Could you check a few things on this model? Use its own coordinates, in mm. Face numbers are marked on the shaded views. A direction names the side the tool comes from. Round coordinates to 2 decimals unless told otherwise and drop trailing zeros. Loops run counter-clockwise (first coordinate to the right, second up) from the corner with the lowest first, then second, coordinate; pieces in that order, holes last. Notation, with made-up numbers: (40, 34.5) -> (72, 34.5) arc R26 ccw to (72, 71.5) -> close; hole circle Ø3 at (-27.5, 77). An arc over 180 degrees is marked (long way). One line per item, written item: value.
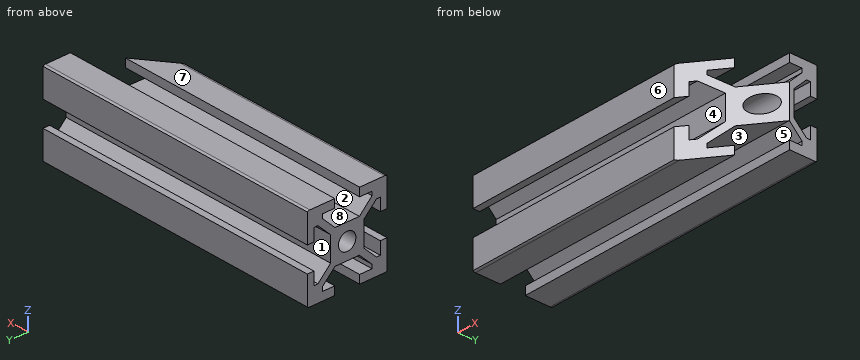
```python
from build123d import *

# Parameters (mm, degrees)
SKETCH1_R                = 2.1
BOSS_EXTRUDE1_DEPTH      = 70
CUT_EXTRUDE_1_DEPTH      = 1
CUT_EXTRUDE_1_DEPTH_BACK = 21


with BuildPart() as part:
    # Sketch1 → Boss-Extrude1 (new body)
    with BuildSketch(Plane(origin=(0, 0, 0), x_dir=(0, 0, -1), z_dir=(1, 0, 0))):
        with BuildLine():
            Line((-10, 9), (-10, 3))
            Line((-10, 3), (-8, 3))
            Line((-8, 3), (-8, 6))
            Line((-8, 6), (-7.060660172, 6))
            Line((-7.060660172, 6), (-4, 2.939339828))
            Line((-4, 2.939339828), (-4, -2.939339828))
            Line((-4, -2.939339828), (-7.060660172, -6))
            Line((-7.060660172, -6), (-8, -6))
            Line((-8, -6), (-8, -3))
            Line((-8, -3), (-10, -3))
            Line((-10, -3), (-10, -9))
            ThreePointArc((-10, -9), (-9.948683298, -9.316227766), (-9.8, -9.6))
            Line((-9.8, -9.6), (-3, -9.6))
            Line((-3, -9.6), (-3, -8))
            Line((-3, -8), (-6, -8))
            Line((-6, -8), (-6, -7.060660172))
            Line((-6, -7.060660172), (-2.939339828, -4))
            Line((-2.939339828, -4), (2.939339828, -4))
            Line((2.939339828, -4), (6, -7.060660172))
            Line((6, -7.060660172), (6, -8))
            Line((6, -8), (3, -8))
            Line((3, -8), (3, -9.6))
            Line((3, -9.6), (9.8, -9.6))
            ThreePointArc((9.8, -9.6), (9.948683298, -9.316227766), (10, -9))
            Line((10, -9), (10, -3))
            Line((10, -3), (8, -3))
            Line((8, -3), (8, -6))
            Line((8, -6), (7.060660172, -6))
            Line((7.060660172, -6), (4, -2.939339828))
            Line((4, -2.939339828), (4, 2.939339828))
            Line((4, 2.939339828), (7.060660172, 6))
            Line((7.060660172, 6), (8, 6))
            Line((8, 6), (8, 3))
            Line((8, 3), (10, 3))
            Line((10, 3), (10, 9))
            ThreePointArc((10, 9), (9.948683298, 9.316227766), (9.8, 9.6))
            Line((9.8, 9.6), (3, 9.6))
            Line((3, 9.6), (3, 8))
            Line((3, 8), (6, 8))
            Line((6, 8), (6, 7.060660172))
            Line((6, 7.060660172), (2.939339828, 4))
            Line((2.939339828, 4), (-2.939339828, 4))
            Line((-2.939339828, 4), (-6, 7.060660172))
            Line((-6, 7.060660172), (-6, 8))
            Line((-6, 8), (-3, 8))
            Line((-3, 8), (-3, 9.6))
            Line((-3, 9.6), (-9.8, 9.6))
            ThreePointArc((-9.8, 9.6), (-9.948683298, 9.316227766), (-10, 9))
        make_face()
        Circle(SKETCH1_R, mode=Mode.SUBTRACT)
    extrude(amount=BOSS_EXTRUDE1_DEPTH)

    # 草图1 → 切除-拉伸1 (cut, two sides)
    with BuildSketch(Plane.XY.offset(10)) as cut_extrude_1_sk:
        Polygon((53.252194875, -9.6), (70, 3), (72.108704706, -2.849693058), (72.521016137, -11.388110896), align=None)
    extrude(amount=CUT_EXTRUDE_1_DEPTH, mode=Mode.SUBTRACT)
    extrude(cut_extrude_1_sk.sketch, amount=-CUT_EXTRUDE_1_DEPTH_BACK, mode=Mode.SUBTRACT)


solid = part.part
```
Item 1: If we section it at D-D on x = 60: Count the separate pieces of the cut face and the enclosed holes in it, plus the area to 3 significant figures.
Output:
separate pieces: 3
enclosed holes: 1
area: 121 mm²
Item 2: If we mould it in two halves opening along Y, with no side actions, what happens to the marked faces 5, 6, 7 and 8? For each: released by +Y, released by -Y, zero draft, split by the parting line, or undercut.
Output:
face 5: undercut
face 6: released by -Y
face 7: zero draft
face 8: undercut
Item 3: Will these pins go through, and if not, where does the flat tip stop? pin 1 Ø1.8 at (x, y) = (44, 1) entering from +Z; pin 2 Ø1 at (x, z) = (27.5, -2) entering from +Y.
Output:
pin 1: stops at z = 4
pin 2: stops at y = 4
Item 4: If we section it at A-A on y = -4.75: List the corners of the cut face in (x, z) for me.
Output:
outline: (0, -10) -> (59.7, -10) -> (59.7, -8) -> (0, -8) -> close; (0, -5.81) -> (59.7, -5.81) -> (59.7, -3.69) -> (0, -3.69) -> close; (0, 3.69) -> (59.7, 3.69) -> (59.7, 5.81) -> (0, 5.81) -> close; (0, 8) -> (59.7, 8) -> (59.7, 10) -> (0, 10) -> close
Item 5: If we section it at B-B on y = 0: List the corners of the cut face in (x, z) for me.
Output:
outline: (0, -4) -> (66.01, -4) -> (66.01, -2.1) -> (0, -2.1) -> close; (0, 2.1) -> (66.01, 2.1) -> (66.01, 4) -> (0, 4) -> close
Item 6: For the marked faces 1, 2, 3 and 4, which set-ups out of +Z, -Z, +X, -X, +Y, -Y let a thin tool reach every point of the face, with its end or its side?
Output:
face 1: +X, -X, +Y
face 2: +X, -X
face 3: -Z, +X, -X
face 4: +X, -X, -Y
Item 7: I need wall thicknesses on line 1 (Z direction, x = 42, y = 0); line 2 (Y direction, x = 50, z = 7.5); line 3 (Z direction, x = 60, y = 5.25). Which ranges of each line are inside material? Lowest first, please. Write a range as from..to.
Output:
line 1: z = -4..-2.1, 2.1..4
line 2: y = -9.6..-6, 6..9.6
line 3: z = -10..-8, -6.31..-4.19, 4.19..6.31, 8..10
Item 8: If we section it at C-C on z = 0: List the corners of the cut face in (x, y) for me.
Output:
outline: (0, -4) -> (60.7, -4) -> (63.22, -2.1) -> (0, -2.1) -> close; (0, 2.1) -> (68.8, 2.1) -> (70, 3) -> (70, 4) -> (0, 4) -> close
